Answer from the drawing. Dimensions are ordinates in mm from the lowest x, y and z of the part. A direction names the side the tool comes from. Round coordinates to 2 decimals unless told otherwise and drop trailing zeros. Write each loop counter-clockwise with the first axis right and the second up, starting at its lowest first coordinate (ties: lowest second). Pieces come first, ordered by that corner, then holes. Notation, with made-up numbers: (-6, -37.5) -> (51, -37.5) arc R36 ccw to (51, -2.5) -> close; hole circle Ø6 at (75.5, 51.25). An arc over 180 degrees is marked (long way). Answer as a JSON object with one key per item and string values. Group by question number.
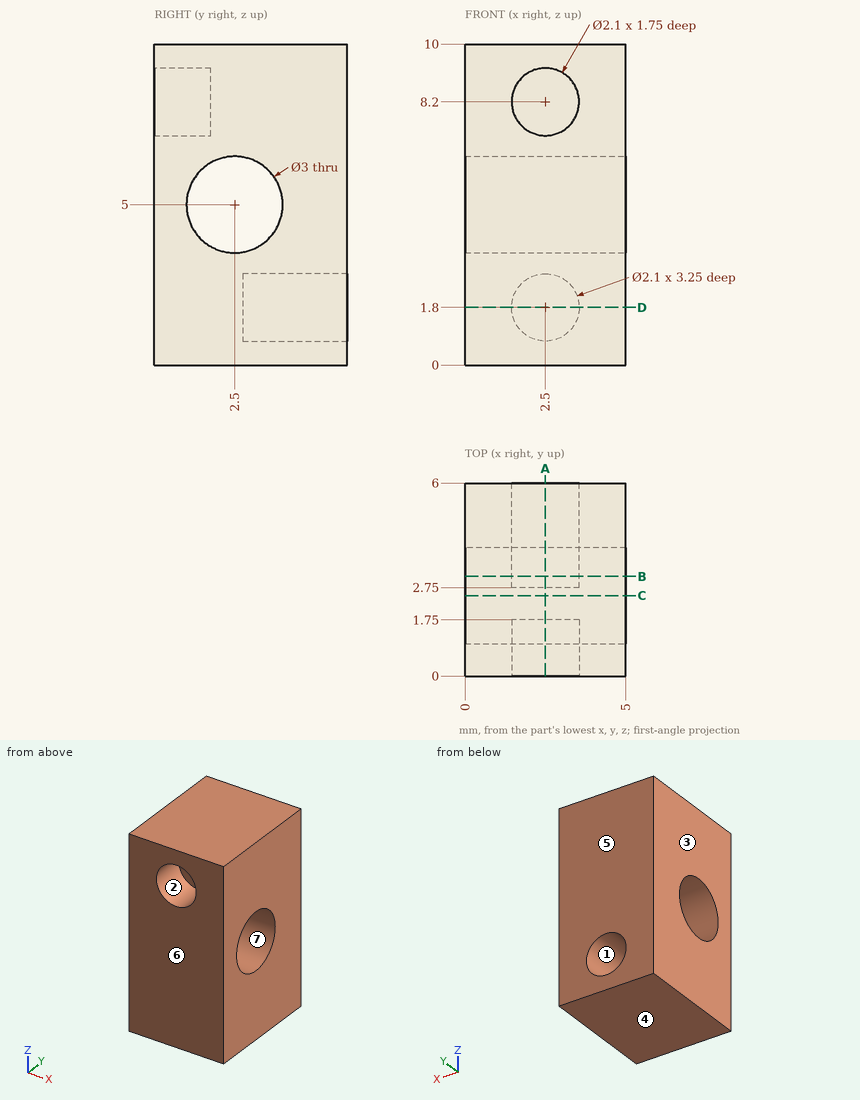
1) A cutting plane is placed at A-A on x = 2.5. Determine the outline of the cut face in (y, z).
2) For a pull along Y with two mould halves and no side action, classify the marked faces 4, 5, 6 and 7 as released by +Y, released by -Y, zero draft, split by the parting line, or undercut.
3) A cutting plane is placed at D-D on z = 1.8. Determine the outline of the cut face in (x, y), plus the area to 3 significant figures.
4) Each of these flat-tipped pins is pushed along its axis until it touches: P1, Ø2.5, axis at y = 2.5, z = 5, coming from the -X side; P2, Ø0.6, axis at x = 3, z = 1.5, coming from the +Y side; P3, Ø0.6, axis at x = 2.5, z = 8.5, coming from the -Y side. Where does it stop, or does it pass through?
5) Straight lines are drawn through the part: L1, parallel to X at y = 3.05, z = 1.75; L2, parallel to Z at x = 3.1, y = 2.5; L3, parallel to Z at x = 2.1, y = 2.9. For each, find the intervals that lie inside material, in ascending order.
6) A cutting plane is placed at C-C on y = 2.5. Determine the outline of the cut face in (x, z), plus the area to 3 significant figures.
7) A cutting plane is placed at B-B on y = 3.1. Determine the outline of the cut face in (x, z), plus the area to 3 significant figures.
8) A tool of negligible diameter and unlimited length cuts with its end or side. For the marked faces 1, 2 and 3, from which of +Z, -Z, +X, -X, +Y, -Y can it reach the whole face along a straight path? Write none if from no direction.
Established:
{
 "1": {"outline": "(0, 0) -> (6, 0) -> (6, 0.75) -> (2.75, 0.75) -> (2.75, 2.85) -> (6, 2.85) -> (6, 10) -> (0, 10) -> (0, 9.25) -> (1.75, 9.25) -> (1.75, 7.15) -> (0, 7.15) -> close; hole circle Ø3 at (2.5, 5)"},
 "2": {"face 4": "zero draft", "face 5": "released by +Y", "face 6": "released by -Y", "face 7": "undercut"},
 "3": {"outline": "(0, 0) -> (5, 0) -> (5, 6) -> (3.55, 6) -> (3.55, 2.75) -> (1.45, 2.75) -> (1.45, 6) -> (0, 6) -> close", "area": "23.2 mm²"},
 "4": {"P1": "passes through", "P2": "stops at y = 2.75", "P3": "stops at y = 1.75"},
 "5": {"L1": "x = 0 to 1.45, 3.55 to 5", "L2": "z = 0 to 3.5, 6.5 to 10", "L3": "z = 0 to 0.83, 2.77 to 3.55, 6.45 to 10"},
 "6": {"outline": "(0, 0) -> (5, 0) -> (5, 3.5) -> (0, 3.5) -> close; (0, 6.5) -> (5, 6.5) -> (5, 10) -> (0, 10) -> close", "area": "35.0 mm²"},
 "7": {"outline": "(0, 0) -> (5, 0) -> (5, 3.63) -> (0, 3.63) -> close; (0, 6.37) -> (5, 6.37) -> (5, 10) -> (0, 10) -> close; hole circle Ø2.1 at (2.5, 1.8)", "area": "32.8 mm²"},
 "8": {"face 1": "+Y", "face 2": "-Y", "face 3": "+Z, -Z, -X, +Y, -Y"}
}
